```python
from build123d import *

# Parameters (mm, degrees)
ESQUISSE1_W                                     = 36
ESQUISSE1_H                                     = 70
BASE_EXTRUSION_DEPTH                            = 14
ESQUISSE10_R                                    = 16
BOSS_EXTRU_3_DEPTH                              = 18
ESQUISSE3_R                                     = 12.5
BOSS_EXTRU_2_DEPTH                              = 5
CHANFREIN1_SIZE                                 = 0.5
CHAMBRAGE_POUR_VIS_T_TE_CYLINDRIQUE_D           = 6.5
CHAMBRAGE_POUR_VIS_T_TE_CYLINDRIQUE_CBORE_D     = 12
CHAMBRAGE_POUR_VIS_T_TE_CYLINDRIQUE_CBORE_DEPTH = 7
R_P_TITION_CIRCULAIRE1_COUNT                    = 4


with BuildPart() as part:
    # Esquisse1 → Base-Extrusion (new body)
    with BuildSketch(Plane(origin=(0, 0, 0), x_dir=(0, 0, -1), z_dir=(1, 0, 0))):
        Rectangle(ESQUISSE1_W, ESQUISSE1_H)
    extrude(amount=-BASE_EXTRUSION_DEPTH)

    # Esquisse10 → Boss.-Extru.3 (add)
    with BuildSketch(Plane.ZY.offset(14)):
        with Locations(Location((0, 0, 0), (0, 0, 180))):
            Circle(ESQUISSE10_R)
    extrude(amount=BOSS_EXTRU_3_DEPTH)

    # Esquisse3 → Boss.-Extru.2 (add)
    with BuildSketch(Plane(origin=(0, 0, 0), x_dir=(0, 0, -1), z_dir=(1, 0, 0))):
        Circle(ESQUISSE3_R)
    extrude(amount=BOSS_EXTRU_2_DEPTH)

    # Chanfrein1
    chanfrein1_edges = [part.edges().sort_by_distance(p)[0] for p in [
        (5, 0, 12.5),
    ]]
    chamfer(chanfrein1_edges, length=CHANFREIN1_SIZE)

    # Chambrage pour vis _ t_te cylindrique (through all)
    with Locations(Plane.ZY.offset(14)):
        with Locations((-7.5, 25), (7.5, 25), (7.252144403, -25), (-7.5, -25)):
            CounterBoreHole(CHAMBRAGE_POUR_VIS_T_TE_CYLINDRIQUE_D / 2, CHAMBRAGE_POUR_VIS_T_TE_CYLINDRIQUE_CBORE_D / 2, CHAMBRAGE_POUR_VIS_T_TE_CYLINDRIQUE_CBORE_DEPTH)

    # Esquisse6 → Enl_vement de mati_re-R_volution1 (revolve, cut)
    with BuildSketch(Plane.XY, mode=Mode.PRIVATE) as enl_vement_de_mati_re_r_volution1_sk:
        Polygon((-32, 1.75), (5, 1.75), (5, 5.5), (-4, 5.5), (-4, 11), (3.5, 11), (3.5, 13.852176113), (8, 13.852176113), (8, 0), (-32, 0), align=None)
    revolve(enl_vement_de_mati_re_r_volution1_sk.sketch.rotate(Axis((0, 0, 0), (1, 0, 0)), 90), axis=Axis((0, 0, 0), (1, 0, 0)), mode=Mode.SUBTRACT)

    # Esquisse8 → Per_age1 (revolve, cut)
    with BuildSketch(Plane(origin=(-32, 0, 0), x_dir=(0, 0, 1), z_dir=(0, 1, 0))):
        Polygon((0, 0), (0, 26.296153426), (7.15, 22), (7.15, 20), (7.278667579, 20), (7.903, 0), align=None)
    revolve(axis=Axis((-38.35, 0, 0), (1, 0, 0)), mode=Mode.SUBTRACT)

    # Esquisse9 → Enl_vement de mati_re-R_volution2 (revolve, cut)
    with BuildSketch(Plane.XY, mode=Mode.PRIVATE) as enl_vement_de_mati_re_r_volution2_sk:
        Polygon((-11.907222504, 4.382957476), (0.437240206, 9.643680185), (1.123318493, 8.033774416), (-11.221144216, 2.773051707), align=None)
    enl_vement_de_mati_re_r_volution2 = revolve(enl_vement_de_mati_re_r_volution2_sk.sketch.rotate(Axis((-35.796822369, -7.700132197, 0), (0.9199461534250014, 0.39204473571079074, 0)), 251.408342684), axis=Axis((-35.796822369, -7.700132197, 0), (0.9199461534250014, 0.39204473571079074, 0)), mode=Mode.SUBTRACT)

    # R_p_tition circulaire1: Enl_vement de mati_re-R_volution2 ×4 about axis
    r_p_tition_circulaire1_axis = Axis((50, 0, 0), (-1, 0, 0))
    for i in range(1, R_P_TITION_CIRCULAIRE1_COUNT):
        add(enl_vement_de_mati_re_r_volution2.rotate(r_p_tition_circulaire1_axis, i * 360 / R_P_TITION_CIRCULAIRE1_COUNT), mode=Mode.SUBTRACT)


solid = part.part
```
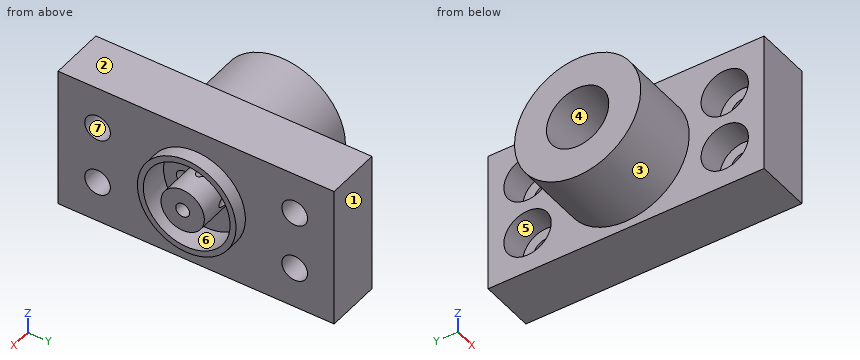
The listing builds one solid part. Answer for the finished solid, in the listing's coordinates (mm). Face numbers are marked on the shaded views. A direction names the side the tool comes from. Coordinates: 2 decimals unless noted, no trailing zeros. Loops run counter-clockwise (first coordinate to the right, second up) from the corner with the lowest first, then second, coordinate; pieces in that order, holes last. Notation, with made-up numbers: M -24,2 L 16,2 A28 cw 16,31 Z; hole C 66,27.5 d3. An arc over 180 degrees is marked long. Answer as a JSON object with one key per item and string values. Group by question number.
Item 1: Determine the mould class of the marked faces 1, 2, 3 and 4 for opening direction Z: +Z half, -Z half, draft (parallel to the pull), parting line (faces both ways), or undercut.
Item 2: Each of these flat-tipped pins is pushed along its axis until it touches: P1, Ø6, axis at y = 25.5, z = 9, coming from the -X side; P2, Ø4, axis at y = -7.5, z = -7.5, coming from the +X side; P3, Ø1, axis at y = 7.5, z = -3.5, coming from the +X side. Where does it stop, or does it pass through?
Item 3: Section C-C (z = 0) is taken. Give the number of separate pieces and of enclosed holes in the cut face, and give its area (3 significant figures).
Item 4: Section A-A (y = 25) is taken. Write down the section's boundary in (x, z), and give its area (3 significant figures).
Item 5: Which of the six approach directions +Z, -Z, +X, -X, +Y, -Y give full straight-line access (tool end or side, diameter ignored) to the marked faces 5, 6 and 7?
Item 6: Consider L1, parallel to Y at x = -3.5, z = 7.5; L2, parallel to Y at x = -11, z = 0; L3, parallel to Y at x = -1.5, z = 0. Determine where each line is inside the solid, lowest interval first.
Item 7: Section B-B (y = -22.5) is taken. Write down the section's boundary in (x, z), and give its area (3 significant figures).
Solved:
{
 "1": {"face 1": "draft", "face 2": "+Z half", "face 3": "parting line", "face 4": "undercut"},
 "2": {"P1": "stops at x = -7", "P2": "stops at x = 3.5", "P3": "stops at x = -4"},
 "3": {"separate pieces": "4", "enclosed holes": "0", "area": "1,140 mm2"},
 "4": {"outline": "M -14,-18 L 0,-18 L 0,-10.75 L -7,-10.75 L -7,-13.5 L -14,-13.5 Z; M -14,-1.5 L -7,-1.5 L -7,-4.25 L 0,-4.25 L 0,4.25 L -7,4.25 L -7,1.5 L -14,1.5 Z; M -14,13.5 L -7,13.5 L -7,10.75 L 0,10.75 L 0,18 L -14,18 Z", "area": "245 mm2"},
 "5": {"face 5": "-X", "face 6": "+X", "face 7": "+X, -X"},
 "6": {"L1": "y = -35 to -28.24, -21.76 to -8.05, 8.05 to 21.75, 28.25 to 35", "L2": "y = -35 to -7.15, 7.15 to 35", "L3": "y = -35 to -11, -5.01 to -1.75, 1.75 to 5.01, 11 to 35"},
 "7": {"outline": "M -14,-18 L 0,-18 L 0,-9.58 L -7,-9.58 L -7,-12.95 L -14,-12.95 Z; M -14,-2.05 L -7,-2.05 L -7,-5.42 L 0,-5.42 L 0,5.18 L -7,5.18 L -7,1.8 L -14,1.8 Z; M -14,12.71 L -7,12.71 L -7,9.33 L 0,9.33 L 0,18 L -14,18 Z", "area": "293 mm2"}
}
